from build123d import *

# Parameters (mm, degrees)
SALIENTE_EXTRUIR1_DEPTH      = 110
SALIENTE_EXTRUIR1_DEPTH_BACK = 10
CROQUIS2_R                   = 45
CORTAR_EXTRUIR1_DEPTH        = 100
CROQUIS3_R                   = 45
CORTAR_EXTRUIR2_DEPTH        = 100
FILLET1_R                    = 60


with BuildPart() as part:
    # Croquis1 → Saliente-Extruir1 (new, two sides: drawn at the far end of the back side and taken through both)
    with BuildSketch(Plane.XY.offset(-SALIENTE_EXTRUIR1_DEPTH_BACK)):
        Polygon((-306.989624487, 145.009245926), (-239.370702608, 0), (0, 0), (0, 210), (-10, 210), (-10, 10), (-233, 10), (-297.926546616, 149.235428543), align=None)
    extrude(amount=SALIENTE_EXTRUIR1_DEPTH + SALIENTE_EXTRUIR1_DEPTH_BACK)

    # Croquis2 → Cortar-Extruir1 (cut)
    with BuildSketch(Plane.ZY.offset(10)):
        with Locations((50, 136.841249694)):
            Circle(CROQUIS2_R)
    extrude(amount=-CORTAR_EXTRUIR1_DEPTH, mode=Mode.SUBTRACT)

    # Croquis3 → Cortar-Extruir2 (cut)
    with BuildSketch(Plane(origin=(-187.554534313, -87.458115672, 0), x_dir=(0, 0, -1), z_dir=(0.906307787036651, 0.4226182617406971, 0))):
        with Locations(Location((-50, 184.347781552, 0), (0, 0, 90))):
            Circle(CROQUIS3_R)
    extrude(amount=-CORTAR_EXTRUIR2_DEPTH, mode=Mode.SUBTRACT)

    # Fillet1
    fillet1_edges = [part.edges().sort_by_distance(p)[0] for p in [
        (-5, 210, 110),
        (-5, 210, -10),
        (-302.458085551, 147.122337235, -10),
        (-302.458085551, 147.122337235, 110),
    ]]
    fillet(fillet1_edges, radius=FILLET1_R - 0.0001)  # a hair under: the kernel refuses the full size


solid = part.part
Design review of the part built by this model. Coordinates are the model's own, in mm. A direction names the side the tool comes from. Give positions to 0.01 mm unless a question says otherwise; leave off trailing zeros. Loops run counter-clockwise (first coordinate to the right, second up) from the corner with the lowest first, then second, coordinate; pieces in that order, holes last. Notation, with made-up numbers: M 47,23 L 95,23 A4 cw 95,28 Z; hole C 63.25,-19.75 d2. An arc over 180 degrees is marked long. One line per question, with ' | ' between items. Start each with the question number.
1. Add section A-A (z = 17.5). Write out the cut boundary in (x, y), plus the area to 3 significant figures.
2. For faces 1 (the face through (-5.07, 191.96, 92.89)), 2 (the face through (-10, 89, 49)), list the 3-axis set-ups (+Z, -Z, +X, -X, +Y, -Y) from which the entire face can be reached by the end or side of a thin tool; tool diameter is ignored.
3. Add section C-C (x = -112). Write out the cut boundary in (y, z), plus the area to 3 significant figures.
4. Insertion check: P1, Ø6, axis at x = -111.5, z = 34.5, coming from the +Y side; P2, Ø5, axis at x = -111, z = 36.5, coming from the -Y side; P3, Ø1, axis at y = 117.5, z = 78, coming from the +X side. Each pin has a flat end and moves straight along its axis. Give the tip position at first contact, or say it passes through.
5. To check wall thickness, follow L1, parallel to Y at x = -4, z = 50; L2, parallel to Y at x = -147, z = 82; L3, parallel to X at y = 40.5, z = 103. State the ranges of each line that lie inside material, in increasing order.
6. Add section B-B (y = 21.5). Write out the cut boundary in (x, z), plus the area to 3 significant figures.
7. The part is to be moulded in two halves that separate along Y. For faces 3 (the face through (-243.367, 32.231, 49.16)), 4 (the face through (-258.63, 41.3, 22.49)), 5 (the face through (-5.07, 181.46, 44.14)), say which applies: released by +Y, released by -Y, zero draft, split by the parting line, or undercut.
8. Add section D-D (z = 33.5). Write out the cut boundary in (x, y), plus the area to 3 significant figures.
Worked out:
1) outline: M -302.95,136.34 L -287.68,103.6 L -278.62,107.83 L -293.88,140.57 Z; M -261.37,47.18 L -239.37,0 L 0,0 L 0,105.72 L -10,105.72 L -10,10 L -233,10 L -252.31,51.41 Z; M -10,167.97 L 0,167.97 L 0,200.44 L -10,200.44 Z | area: 4,490 mm²
2) face 1: +Z, +X, -X, +Y | face 2: +Z, -Z, +Y
3) outline: M 0,-10 L 10,-10 L 10,110 L 0,110 Z | area: 1,200 mm²
4) P1: stops at y = 10 | P2: stops at y = 0 | P3: stops at x = -282.89
5) L1: y = 0 to 91.84, 181.84 to 210 | L2: y = 0 to 10 | L3: x = -258.26 to -247.22, -10 to 0
6) outline: M -249.4,-10 L -238.36,-10 L -238.36,110 L -249.4,110 Z; M -10,-10 L 0,-10 L 0,110 L -10,110 Z | area: 2,520 mm²
7) face 3: released by +Y | face 4: released by -Y | face 5: undercut
8) outline: M -306.01,142.91 L -292.22,113.33 L -283.16,117.56 L -296.95,147.14 Z; M -256.83,37.45 L -239.37,0 L 0,0 L 0,94.98 L -10,94.98 L -10,10 L -233,10 L -247.77,41.67 Z; M -10,178.71 L 0,178.71 L 0,207.69 L -10,207.69 Z | area: 4,210 mm²
